Can you work these out from the drawing? Everything is in mm from the part's minimum corner. Give positions to 0.01 mm unless a question says otherwise; leave off trailing zeros. Write each loop counter-clockwise with the first axis right and the second up, starting at its lowest first coordinate (ties: lowest second). Pieces come first, ordered by that corner, then holes. Notation, with made-up numbers: (43, 12) -> (95, 12) arc R24 cw to (95, 51) -> close; hole circle Ø3 at (72, -40). An arc over 180 degrees is marked (long way). Use one line per item in the form item = value.
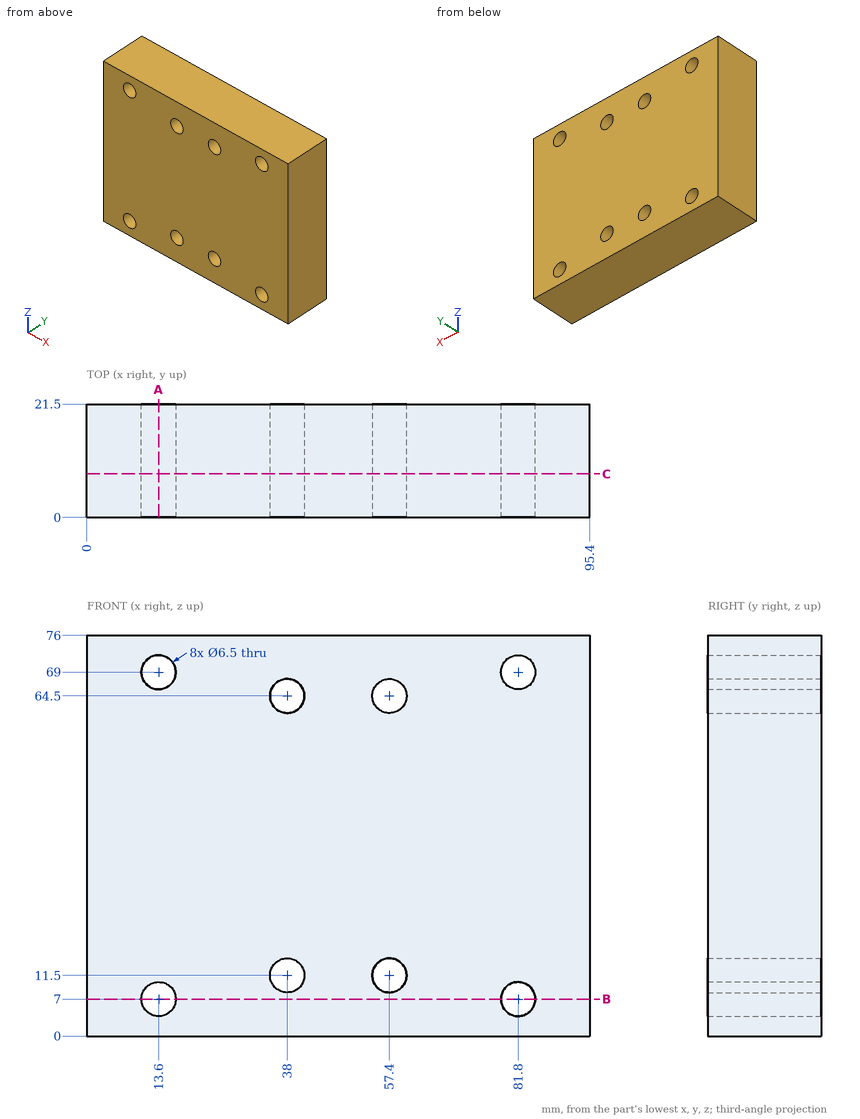
Q1. I want a section at A-A, the plane x = 13.6. Write out the boundary of the cut face in (y, z).
Result set:
outline = (0, 0) -> (21.5, 0) -> (21.5, 3.75) -> (0, 3.75) -> close; (0, 10.25) -> (21.5, 10.25) -> (21.5, 65.75) -> (0, 65.75) -> close; (0, 72.25) -> (21.5, 72.25) -> (21.5, 76) -> (0, 76) -> close
Q2. Will this pin go through, and if not, where does the flat tip stop? pin 1 Ø3 at (x, y) = (50, 17) entering from -Z.
Result set:
pin_1 = 0
Q3. If I drill on line 1 along X through (y, z) = (16.25, 11.5); line 2 along Z through (x, y) = (81.8, 6.25); line 3 along Z through (x, y) = (38, 12), over which ranges is the centre line in solid material (lowest first)? Write a range as from..to.
Result set:
line_1 = 0..34.75, 41.25..54.15, 60.65..95.4
line_2 = 0..3.75, 10.25..65.75, 72.25..76
line_3 = 0..8.25, 14.75..61.25, 67.75..76
Q4. I want a section at C-C, the plane y = 8.25. Count the separate pieces of the cut face and the enclosed holes in it, and give its area (3 significant figures).
Result set:
separate_pieces = 1
enclosed_holes = 8
area = 6,980 mm2
Q5. I want a section at B-B, the plane z = 7. Write out the boundary of the cut face in (x, y), and give its area (3 significant figures).
Result set:
outline = (0, 0) -> (10.35, 0) -> (10.35, 21.5) -> (0, 21.5) -> close; (16.85, 0) -> (78.55, 0) -> (78.55, 21.5) -> (16.85, 21.5) -> close; (85.05, 0) -> (95.4, 0) -> (95.4, 21.5) -> (85.05, 21.5) -> close
area = 1,770 mm2
